Here's the drawing with two shaded views (mm, measured from the low corner). I have some questions. A direction names the side the tool comes from. Give positions to 0.01 mm unless a question says otherwise; leave off trailing zeros. Loops run counter-clockwise (first coordinate to the right, second up) from the corner with the lowest first, then second, coordinate; pieces in that order, holes last. Notation, with made-up numbers: (16, -6) - (34, -6) arc R14 cw to (34, 10) - close; hole circle Ø2 at (-15.5, 10.25). An arc over 180 degrees is marked (long way). Use one line per item in the form item = value.
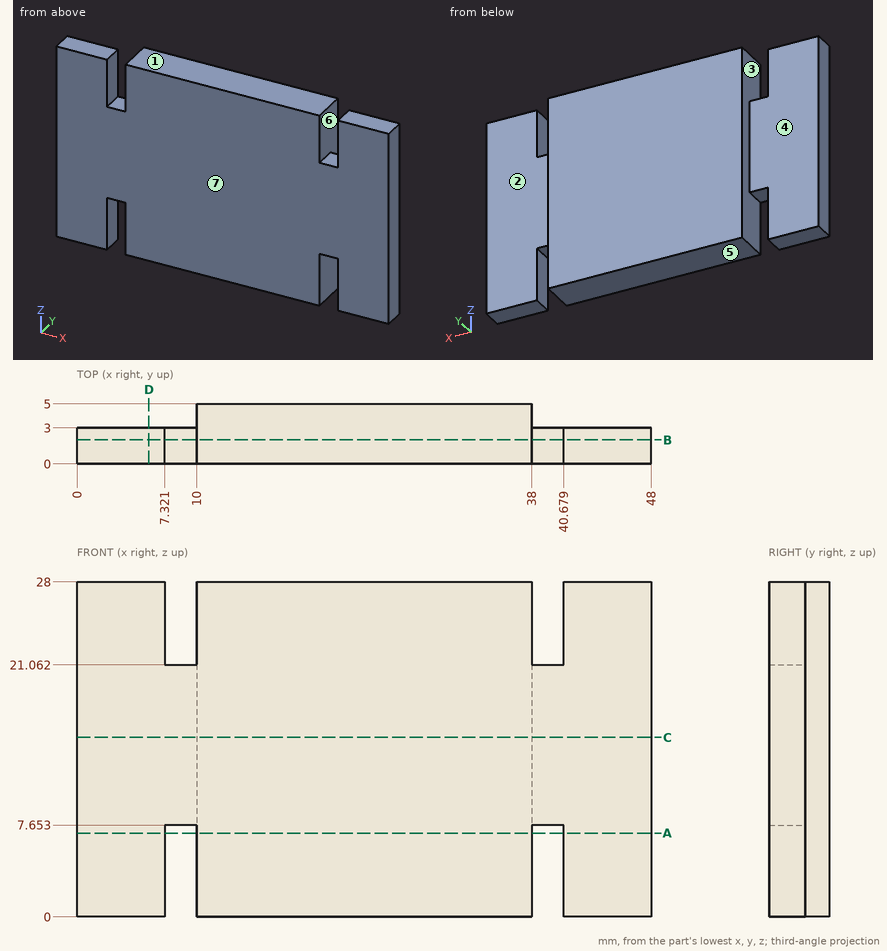
(1) If we section it at A-A (z = 7): List the corners of the cut face in (x, y) for me.
Geometry says:
outline = (0, 0) - (7.32, 0) - (7.32, 3) - (0, 3) - close; (10, 0) - (38, 0) - (38, 5) - (10, 5) - close; (40.68, 0) - (48, 0) - (48, 3) - (40.68, 3) - close
(2) If I drill on probe 1 along X at (y, z) = (2.95, 7); probe 2 along Y at (x, z) = (2, 4.25); probe 3 along X at (y, z) = (4, 4.5), over which ranges is the centre line in solid material (lowest first)?
Geometry says:
probe_1 = 0 to 7.32, 10 to 38, 40.68 to 48
probe_2 = 0 to 3
probe_3 = 10 to 38
(3) If we section it at D-D (x = 6): List the corners of the cut face in (y, z) for me.
Geometry says:
outline = (0, 0) - (3, 0) - (3, 28) - (0, 28) - close
(4) If we section it at C-C (z = 15): List the corners of the cut face in (x, y) for me, plus the area to 3 significant figures.
Geometry says:
outline = (0, 0) - (48, 0) - (48, 3) - (38, 3) - (38, 5) - (10, 5) - (10, 3) - (0, 3) - close
area = 200 mm²
(5) For the marked faces 1, 2, 3, 4 and 5, which set-ups out of +Z, -Z, +X, -X, +Y, -Y let a thin tool reach every point of the face, with its end or its side?
Geometry says:
face_1 = +Z, +X, -X, +Y, -Y
face_2 = +Z, -Z, +X, +Y
face_3 = +Y
face_4 = +Z, -Z, -X, +Y
face_5 = -Z, +X, -X, +Y, -Y
(6) If we section it at B-B (y = 2): List the corners of the cut face in (x, z) for me, plus the area to 3 significant figures.
Geometry says:
outline = (0, 0) - (7.32, 0) - (7.32, 7.65) - (10, 7.65) - (10, 0) - (38, 0) - (38, 7.65) - (40.68, 7.65) - (40.68, 0) - (48, 0) - (48, 28) - (40.68, 28) - (40.68, 21.06) - (38, 21.06) - (38, 28) - (10, 28) - (10, 21.06) - (7.32, 21.06) - (7.32, 28) - (0, 28) - close
area = 1,270 mm²
(7) For P1, Ø1.5, axis at y = 2, z = 2, coming from the -X side; P2, Ø0.8, axis at x = 8.5, y = 1, coming from the -Z side; P3, Ø3, axis at x = 5.5, z = 20, coming from the +Y side; P4, Ø1.3, axis at x = 8.5, y = 2, coming from the +Z side, each with a flat end and sliding along its axis, tell me the tip position at first contact or that it passes through.
Geometry says:
P1 = 0
P2 = 7.65
P3 = 3
P4 = 21.06
(8) Thinking about a two-plate mould opening in X: for the marked faces 6 and 7, which applies, pulls with the +X half, pulls with the -X half, needs draft (parallel to the pull), parting line crosses it, or undercut?
Geometry says:
face_6 = undercut
face_7 = needs draft
